Check sheet for the modelled part. Datum: model origin and axes. Units: mm. A direction names the side the tool comes from. Round coordinates to 2 decimals unless told otherwise and drop trailing zeros. Loops run counter-clockwise (first coordinate to the right, second up) from the corner with the lowest first, then second, coordinate; pieces in that order, holes last. Notation, with made-up numbers: (-20.75, -10.75) - (-0.75, -10.75) arc R24 cw to (-0.75, 0.25) - close; hole circle Ø9 at (-25, 55.5). An arc over 180 degrees is marked (long way). Put each result on its own line as item: value.
```python
from build123d import *

# Parameters (mm, degrees)
BOSS_EXTRUDE1_DEPTH = 35
SKETCH2_R           = 3
CUT_EXTRUDE1_DEPTH  = 10


with BuildPart() as part:
    # Sketch1 → Boss-Extrude1 (new, symmetric)
    with BuildSketch(Plane.XY):
        with BuildLine():
            Line((19.4, -38.1), (-19.4, -38.1))
            ThreePointArc((-19.4, -38.1), (-23.642640687, -36.342640687), (-25.4, -32.1))
            Line((-25.4, -32.1), (-25.4, 32.1))
            ThreePointArc((-25.4, 32.1), (-23.642640687, 36.342640687), (-19.4, 38.1))
            Line((-19.4, 38.1), (19.4, 38.1))
            ThreePointArc((19.4, 38.1), (23.642640687, 36.342640687), (25.4, 32.1))
            Line((25.4, 32.1), (25.4, -32.1))
            ThreePointArc((25.4, -32.1), (23.642640687, -36.342640687), (19.4, -38.1))
        make_face()
        with BuildLine():
            Line((19.4, 34.925), (-19.4, 34.925))
            ThreePointArc((-19.4, 34.925), (-21.397576657, 34.097576657), (-22.225, 32.1))
            Line((-22.225, 32.1), (-22.225, -32.1))
            ThreePointArc((-22.225, -32.1), (-21.397576657, -34.097576657), (-19.4, -34.925))
            Line((-19.4, -34.925), (19.4, -34.925))
            ThreePointArc((19.4, -34.925), (21.397576657, -34.097576657), (22.225, -32.1))
            Line((22.225, -32.1), (22.225, 32.1))
            ThreePointArc((22.225, 32.1), (21.397576657, 34.097576657), (19.4, 34.925))
        make_face(mode=Mode.SUBTRACT)
    extrude(amount=BOSS_EXTRUDE1_DEPTH, both=True)

    # Sketch2 → Cut-Extrude1 (cut)
    with BuildSketch(Plane(origin=(25.4, 0, 0), x_dir=(0, 0, -1), z_dir=(1, 0, 0))):
        with Locations(Location((-20, 26.5, 0), (0, 0, 90))):
            Circle(SKETCH2_R)
        with Locations(Location((20, 26.5, 0), (0, 0, 90))):
            Circle(SKETCH2_R)
        with Locations(Location((20, -26.5, 0), (0, 0, 90))):
            Circle(SKETCH2_R)
        with Locations(Location((-20, -26.5, 0), (0, 0, 90))):
            Circle(SKETCH2_R)
    extrude(amount=-CUT_EXTRUDE1_DEPTH, mode=Mode.SUBTRACT)


solid = part.part
```
Item 1: Go/stop test with a flat-tipped pin: pin 1 (5 mm diameter, centred on y = -26.5, z = 20, fed in from +X) (3 decimals). Record where the tip stops, or that it passes through.
Filled sheet:
pin 1: x = -22.225
Item 2: Tool access check on faces 4 (the cylindrical face through (23.8, -28.9, 18.2)), 5 (the cylindrical face through (23.689, -36.296, 0.49)), 6 (the cylindrical face through (21.375, -34.119, 0.49)). Record the directions out of +Z, -Z, +X, -X, +Y, -Y that give a thin tool (end or side, any length) a straight path to the whole face; none if there is none.
Filled sheet:
face 4: +X
face 5: +Z, -Z, +X, -Y
face 6: +Z, -Z
Item 3: Release check for a two-part mould opening along Y. For faces 1 (the flat face through (23, 0, 35)), 2 (the flat face through (0, 34.925, 0)), 3 (the cylindrical face through (-23.689, 36.296, 0.49)) record: +Y half, -Y half, draft (parallel to the pull), parting line (faces both ways), or undercut.
Filled sheet:
face 1: draft
face 2: undercut
face 3: +Y half
Item 4: Section check A-A on y = 26.5. Enter the section's corners in (x, z) (3 decimals).
Filled sheet:
outline: (-25.4, -35) - (-22.225, -35) - (-22.225, 35) - (-25.4, 35) - close; (22.225, -35) - (25.4, -35) - (25.4, -23) - (22.225, -23) - close; (22.225, -17) - (25.4, -17) - (25.4, 17) - (22.225, 17) - close; (22.225, 23) - (25.4, 23) - (25.4, 35) - (22.225, 35) - close
Item 5: Section check C-C on z = -8. Enter the section's corners in (x, y) (3 decimals), then the cut area to 3 significant figures.
Filled sheet:
outline: (-25.4, -32.1) arc R6 ccw to (-19.4, -38.1) - (19.4, -38.1) arc R6 ccw to (25.4, -32.1) - (25.4, 32.1) arc R6 ccw to (19.4, 38.1) - (-19.4, 38.1) arc R6 ccw to (-25.4, 32.1) - close; hole (-22.225, -32.1) arc R2.825 ccw to (-19.4, -34.925) - (19.4, -34.925) arc R2.825 ccw to (22.225, -32.1) - (22.225, 32.1) arc R2.825 ccw to (19.4, 34.925) - (-19.4, 34.925) arc R2.825 ccw to (-22.225, 32.1) - close
area: 742 mm²
Item 6: Section check B-B on x = 10. Enter the section's corners in (y, z) (3 decimals).
Filled sheet:
outline: (-38.1, -35) - (-34.925, -35) - (-34.925, 35) - (-38.1, 35) - close; (34.925, -35) - (38.1, -35) - (38.1, 35) - (34.925, 35) - close
Item 7: Section check D-D on z = -20. Enter the section's corners in (x, y) (3 decimals), then the cut area to 3 significant figures.
Filled sheet:
outline: (-25.4, -32.1) arc R6 ccw to (-19.4, -38.1) - (19.4, -38.1) arc R6 ccw to (25.4, -32.1) - (25.4, -29.5) - (22.225, -29.5) - (22.225, -32.1) arc R2.825 cw to (19.4, -34.925) - (-19.4, -34.925) arc R2.825 cw to (-22.225, -32.1) - (-22.225, 32.1) arc R2.825 cw to (-19.4, 34.925) - (19.4, 34.925) arc R2.825 cw to (22.225, 32.1) - (22.225, 29.5) - (25.4, 29.5) - (25.4, 32.1) arc R6 ccw to (19.4, 38.1) - (-19.4, 38.1) arc R6 ccw to (-25.4, 32.1) - close; (22.225, -23.5) - (25.4, -23.5) - (25.4, 23.5) - (22.225, 23.5) - close
area: 704 mm²
Item 8: Thickness scan on line 1 (Z direction, x = 24.1, y = -26.5); line 2 (X direction, y = 30.5, z = 13) (3 decimals); line 3 (Y direction, x = -1.5, z = 24) (3 decimals). Record the ranges inside material, lowest first. Write a range as from..to.
Filled sheet:
line 1: -35..-23, -17..17, 23..35
line 2: -25.4..-22.225, 22.225..25.4
line 3: -38.1..-34.925, 34.925..38.1
